```python
from build123d import *

# Parameters (mm, degrees)
F0_W      = 1
F0_H      = 2.5
F0_H_2    = 1.5
F1_DEPTH  = 10
F3_W      = 4
F3_H      = 2.7
F3_W_2    = 1
F4_DEPTH  = 7
F6_DEPTH  = 7.3
F7_DEPTH  = 1
F8_DEPTH  = 0.5
F9_DEPTH  = 0.5
F10_DEPTH = 0.5
F11_W     = 2
F11_H     = 14.978
F12_DEPTH = 25
F13_DEPTH = 1.2
F14_R     = 1.5


with BuildPart() as f1:
    # F0 (on Front) → F1 (new body)
    with BuildSketch(Plane.XZ):
        with BuildLine():
            Line((0, 2.5), (0, 0))
            Line((0, 0), (4, 0))
            Line((4, 0), (4, 1.55))
            Line((4, 1.55), (3.990259403, 1.5685071343))
            ThreePointArc((3.990259403, 1.5685071343), (3.8184891819, 2.0202463599), (3.7600958477, 2.5))
            ThreePointArc((3.7600958477, 2.5), (3.8184891819, 2.9797536401), (3.990259403, 3.4314928657))
            Line((3.990259403, 3.4314928657), (4, 3.45))
            Line((4, 3.45), (4, 4))
            Line((4, 4), (0, 4))
            Line((0, 4), (0, 2.5))
        make_face()
        with Locations((-0.5, 1.25)):
            Rectangle(F0_W, F0_H)
        Polygon((4, 0), (0, 0), (-1, 0), (4, -1.5), align=None)
        with Locations((-0.5, 3.25)):
            Rectangle(F0_W, F0_H_2)
    extrude(amount=F1_DEPTH)

    # F3 (on offset) → F4 (join)
    with BuildSketch(Plane.XY.offset(1)):
        with Locations((2, -1.35)):
            Rectangle(F3_W, F3_H)
        with Locations((-0.5, -1.35)):
            Rectangle(F3_W_2, F3_H)
    extrude(amount=-F4_DEPTH)

    # F5 (on face) → F6 (join, through all)
    with BuildSketch(Plane.XZ.offset(2.7)):
        Polygon((-1, -6), (4, -6), (4, -2.2), (-1, -0.7), align=None)
    extrude(amount=F6_DEPTH)

    # F7 (add): a face of the model
    f7_faces = [f1.faces().sort_by_distance(p)[0] for p in [
        (1.5, -5, -6),
    ]]
    extrude(f7_faces, amount=F7_DEPTH)

    # F8 (add): a face of the model
    f8_faces = [f1.faces().sort_by_distance(p)[0] for p in [
        (1.5, -5, 4),
    ]]
    extrude(f8_faces, amount=F8_DEPTH)

    # F9 (cut): a face of the model
    f9_faces = [f1.faces().sort_by_distance(p)[0] for p in [
        (1.4870709663, 0, -1.2701719647),
    ]]
    extrude(f9_faces, amount=-F9_DEPTH, mode=Mode.SUBTRACT)

    # F10 (add): a face of the model
    f10_faces = [f1.faces().sort_by_distance(p)[0] for p in [
        (1.5, -5.25, 4.5),
    ]]
    extrude(f10_faces, amount=F10_DEPTH)

    # F11 (on face) → F12 (cut)
    with BuildSketch(Plane.XZ.offset(10)):
        with Locations((0, -0.511)):
            Rectangle(F11_W, F11_H)
    extrude(amount=-F12_DEPTH, mode=Mode.SUBTRACT)

    # F13 (add): a face of the model
    f13_faces = [f1.faces().sort_by_distance(p)[0] for p in [
        (2.5, -5.25, 5),
    ]]
    extrude(f13_faces, amount=F13_DEPTH)

    # F14
    f14_edges = [f1.edges().sort_by_distance(p)[0] for p in [
        (2.5, -10, 6.2),
        (2.5, -0.5, 6.2),
    ]]
    fillet(f14_edges, radius=F14_R)


with BuildPart() as f16_1:
    # F16: instance of F1
    add(f1.part.mirror(Plane(origin=(2.5, -5.25, -8), x_dir=(1, 0, 0), z_dir=(0, 0, -1))))


solid = f16_1.part
```
The listing builds one solid part. Answer for the finished solid, in the listing's coordinates (mm). A direction names the side the tool comes from. Round coordinates to 2 decimals unless told otherwise and drop trailing zeros. Write each loop counter-clockwise with the first axis right and the second up, starting at its lowest first coordinate (ties: lowest second). Pieces come first, ordered by that corner, then holes. Notation, with made-up numbers: (-27, 82.5) -> (5, 82.5) arc R23 ccw to (5, 109.5) -> close; hole circle Ø4 at (17.25, -25.5). An arc over 180 degrees is marked (long way). Use CSV: the item, a comma, the result in double quotes. Start each with the question number.
(1) The mould has two halves that part along X. Classify faces 1 (the face through (4, -5, -13)), 2 (the face through (2.521, -6.299, -14.244)), 3 (the face through (2.5, -2.7, -14.6)), 4 (the face through (2, -10, -12)): released by +X, released by -X, zero draft, split by the parting line, or undercut.
(2) Consider L1, parallel to Z at x = 1.7, y = -6.75; L2, parallel to Z at x = 1.25, y = -7 (3 decimals); L3, parallel to Y at x = 2.8, z = -14.5. Determine where each line is inside the solid, lowest interval first. Write a range as from..to.
(3) Section D-D on z = -18.75 is taken. Give the vertices of the cut face in (x, y), then the cut area to 3 significant figures.
(4) Section B-B on x = 2 is taken. Give the vertices of the cut face in (y, z).
(5) Which of the six approach directions +Z, -Z, +X, -X, +Y, -Y give full straight-line access (tool end or side, diameter ignored) to faces 5 (the face through (2.48, -0.93, -21.75)), 6 (the face through (2.479, -6.299, -14.956))?
(6) Section C-C on z = -14.25 is taken. Give the vertices of the cut face in (x, y), then the cut area to 4 significant figures.
A:
1,face 1,"released by +X"
1,face 2,"undercut"
1,face 3,"undercut"
1,face 4,"zero draft"
2,L1,"z = -22.2..-15.19, -14.49..-9"
2,L2,"z = -22.2..-15.325, -14.625..-9"
2,L3,"y = -2.7..-0.5"
3,outline,"(1, -10) -> (3.78, -10) -> (3.78, -0.5) -> (1, -0.5) -> close"
3,area,"26.4 mm²"
4,outline,"(-10, -20.7) arc R1.5 ccw to (-8.5, -22.2) -> (-2, -22.2) arc R1.5 ccw to (-0.5, -20.7) -> (-0.5, -9) -> (-10, -9) -> (-10, -14.4) -> (-2.7, -14.4) -> (-2.7, -15.1) -> (-10, -15.1) -> close"
5,face 5,"-Z, +X, -X, +Y"
5,face 6,"-Y"
6,outline,"(1, -10) -> (2.5, -10) -> (2.5, -2.7) -> (4, -2.7) -> (4, -0.5) -> (1, -0.5) -> close"
6,area,"17.55 mm²"
